```python
from build123d import *

# Parameters (mm, degrees)
SKETCH2_R           = 1.2
BOSS_EXTRUDE1_DEPTH = 4
FILLET1_R           = 5


with BuildPart() as part:
    # Sketch2 → Boss-Extrude1 (new body)
    with BuildSketch(Plane.XY):
        with BuildLine():
            Line((0, 4), (0, 0))
            Line((0, 0), (38.9, 0))
            Line((38.9, 0), (38.9, 4))
            Line((38.9, 4), (34.9, 4))
            Line((34.9, 4), (34.9, 7.5))
            Line((34.9, 7.5), (30.9, 7.5))
            Line((30.9, 7.5), (30.9, 11.5))
            Line((30.9, 11.5), (32.029872408, 11.5))
            ThreePointArc((32.029872408, 11.5), (33.95, 21.5), (32.029872408, 31.5))
            Line((32.029872408, 31.5), (16.95, 31.5))
            ThreePointArc((16.95, 31.5), (-3.05, 31.5), (-3.05, 11.5))
            Line((-3.05, 11.5), (8, 11.5))
            Line((8, 11.5), (8, 7.5))
            Line((8, 7.5), (4, 7.5))
            Line((4, 7.5), (4, 4))
            Line((4, 4), (0, 4))
        make_face()
        with BuildLine():
            ThreePointArc((12.472095652, 24.340873036), (15.55, 21.5), (12.472095652, 18.659126964))
            ThreePointArc((12.472095652, 18.659126964), (0.74, 21.5), (12.472095652, 24.340873036))
        make_face(mode=Mode.SUBTRACT)
        with Locations((29.16, 21.5)):
            Circle(SKETCH2_R, mode=Mode.SUBTRACT)
    extrude(amount=BOSS_EXTRUDE1_DEPTH)

    # Fillet1
    fillet1_edges = [part.edges().sort_by_distance(p)[0] for p in [
        (16.95, 31.5, 2),
        (32.029872408, 31.5, 2),
    ]]
    fillet(fillet1_edges, radius=FILLET1_R)


solid = part.part
```
Geometry: final body of the model. Coordinates: model frame, mm. A direction names the side the tool comes from. Give positions to 0.01 mm unless a question says otherwise; leave off trailing zeros. Order: outer loops, then holes, each group sorted by start corner. A loop starts at its lowest first (then second) coordinate and runs counter-clockwise, first axis right, second up. Notation, with made-up numbers: M -26.5,81.5 L -8.5,81.5 A18 ccw -8.5,85.5 Z; hole C -2,37 d1. An arc over 180 degrees is marked long. Answer as CSV lines item,"result". Start each with the question number.
1) Cut plane C-C (z = 1.7). Output: boundary loops of the cut face in (x, y).
2) Set-up query: faces 5 (the flat face through (33, 7.5, 2)), 6 (the flat face through (37, 4, 2)), 7 (the flat face through (4, 6, 2)). Return all of +Z, -Z, +X, -X, +Y, -Y with unobstructed straight access to the full face (end or side cutting, diameter ignored); none if empty.
3) Cut plane A-A (x = 6.95). Output: boundary loops of the cut face in (y, z).
4) Mould query, pull axis X, two halves, no side actions, for faces 1 (the cylindrical face through (0.744, 21.268, 1.972)), 2 (the flat face through (8, 10, 2)), 3 (the cylindrical face through (33.865, 19.36, 1.972)), 4 (the flat face through (24, 31.5, 2)). Classes: +X half, -X half, draft (parallel to the pull), parting line (faces both ways), or undercut.
5) Cut plane D-D (x = 29.16). Output: boundary loops of the cut face in (y, z), then the cut area to 3 significant figures.
6) Cut plane B-B (y = 21.5). Output: boundary loops of the cut face in (x, z).
7) First-contact query: P1, Ø2, axis at x = 22, z = 2.5, coming from the +Y side; P2, Ø1.2, axis at x = 33.5, z = 1.5, coming from the +Y side; P3, Ø1.2, axis at y = 1.5, z = 1.5, coming from the -X side; P4, Ø1.9, axis at x = 29.16, y = 21.5, coming from the +Z side. Flat tips, straight axial feed; report the tip coordinate or a pass-through.
8) Line query: line 1 (Y direction, x = 6.95, z = 1.1); line 2 (X direction, y = 22, z = 0.3); line 3 (X direction, y = 8, z = 2.6). Output: solid intervals per line, ascending. Write a range as from..to.
Findings below:
1,outline,"M -3.05,11.5 L 8,11.5 L 8,7.5 L 4,7.5 L 4,4 L 0,4 L 0,0 L 38.9,0 L 38.9,4 L 34.9,4 L 34.9,7.5 L 30.9,7.5 L 30.9,11.5 L 32.03,11.5 A27 ccw 33.24,27.64 A5 ccw 28.37,31.5 L 18.84,31.5 A5 cw 15.74,32.58 A14.14 ccw Z; hole M 12.47,18.66 A2.85 ccw long 12.47,24.34 A6.21 ccw long Z; hole C 29.16,21.5 d2.4"
2,face 5,"+Z, -Z, +X"
2,face 6,"+Z, -Z, +X, +Y"
2,face 7,"+Z, -Z, -X"
3,outline,"M 0,0 L 7.5,0 L 7.5,4 L 0,4 Z; M 11.5,0 L 15.29,0 L 15.29,4 L 11.5,4 Z; M 27.71,0 L 35.64,0 L 35.64,4 L 27.71,4 Z"
4,face 1,"undercut"
4,face 2,"-X half"
4,face 3,"+X half"
4,face 4,"draft"
5,outline,"M 0,0 L 20.3,0 L 20.3,4 L 0,4 Z; M 22.7,0 L 31.44,0 L 31.44,4 L 22.7,4 Z"
5,area,"116 mm²"
6,outline,"M -7.19,0 L 0.74,0 L 0.74,4 L -7.19,4 Z; M 15.55,0 L 27.96,0 L 27.96,4 L 15.55,4 Z; M 30.36,0 L 33.95,0 L 33.95,4 L 30.36,4 Z"
7,P1,"stops at y = 31.5"
7,P2,"stops at y = 28.63"
7,P3,"stops at x = 0"
7,P4,"passes through"
8,line 1,"y = 0..7.5, 11.5..15.29, 27.71..35.64"
8,line 2,"x = -7.18..0.76, 15.51..28.07, 30.25..33.95"
8,line 3,"x = 8..30.9"
